Design review of the part shown in the three views and the two pictorial views. Dimensions are in mm from the part's minimum x, y and z. Give positions to 0.01 mm unless a question says otherwise; leave off trailing zeros. Order: outer loops, then holes, each group sorted by start corner. A loop starts at its lowest first (then second) coordinate and runs counter-clockwise, first axis right, second up.
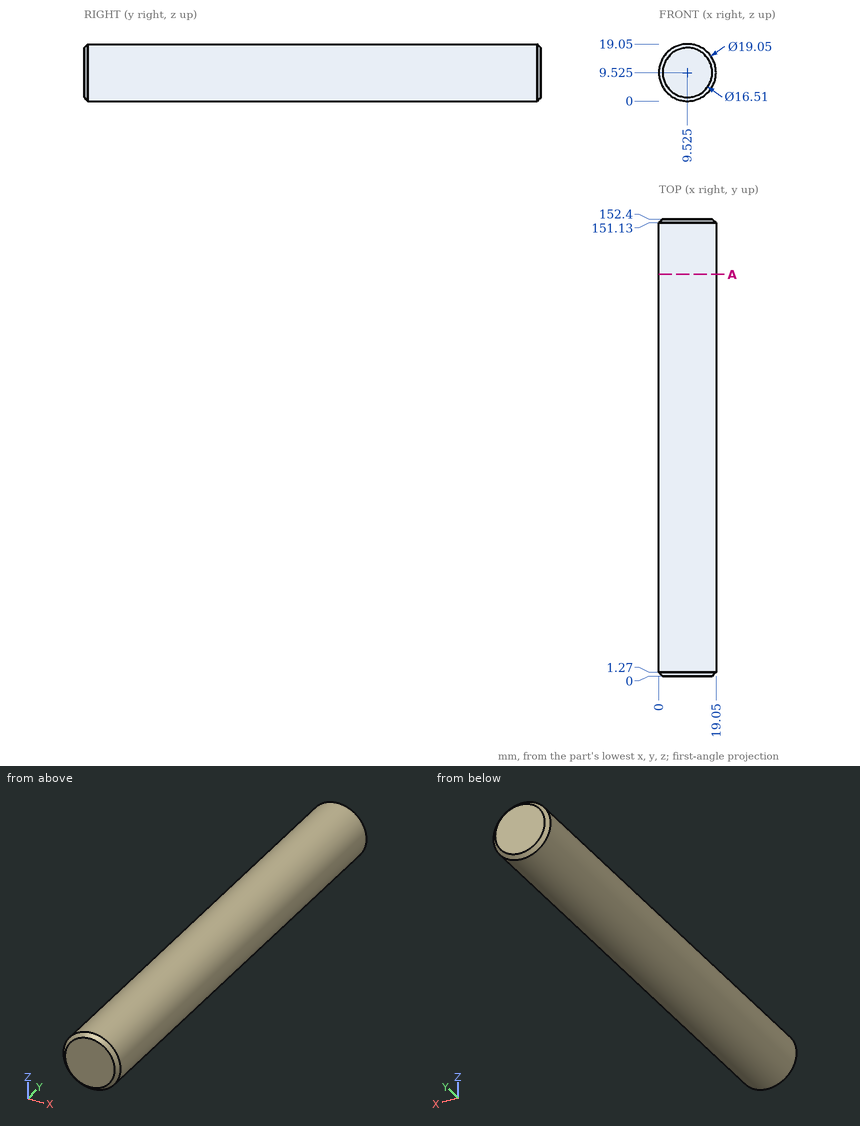
Item 1: Clearance check with flat-ended pins moving along their axes: pin 1 Ø1.5 at (x, y) = (6.5, 16.5) entering from +Z; pin 2 Ø8 at (x, y) = (2.5, 113) entering from -Z; pin 3 Ø1.5 at (y, z) = (55.5, 15) entering from -X; pin 4 Ø1.5 at (x, y) = (10, 102.5) entering from -Z. State where each tip first meets the part, or that it passes through.
Values found:
pin 1: stops at z = 18.77
pin 2: stops at z = 0.49
pin 3: stops at x = 1.25
pin 4: stops at z = 0
Item 2: Take a section at A-A (y = 134). Give the boundary of the cut face in (x, z) (3 decimals).
Values found:
outline: circle Ø19.05 at (9.525, 9.525)
Item 3: For line 1 (X direction, y = 94, z = 14.25); line 2 (Z direction, x = 10.25, y = 89); line 3 (Z direction, x = 4.75, y = 107.5), list the stretches that pass through material, from the lowest coordinate up.
Values found:
line 1: x = 1.25 to 17.8
line 2: z = 0.03 to 19.02
line 3: z = 1.28 to 17.77
